Could you check a few things on this drawing? It's one solid part, dimensions in mm from its lowest x, y, z. A direction names the side the tool comes from. Give positions to 0.01 mm unless a question says otherwise; leave off trailing zeros.
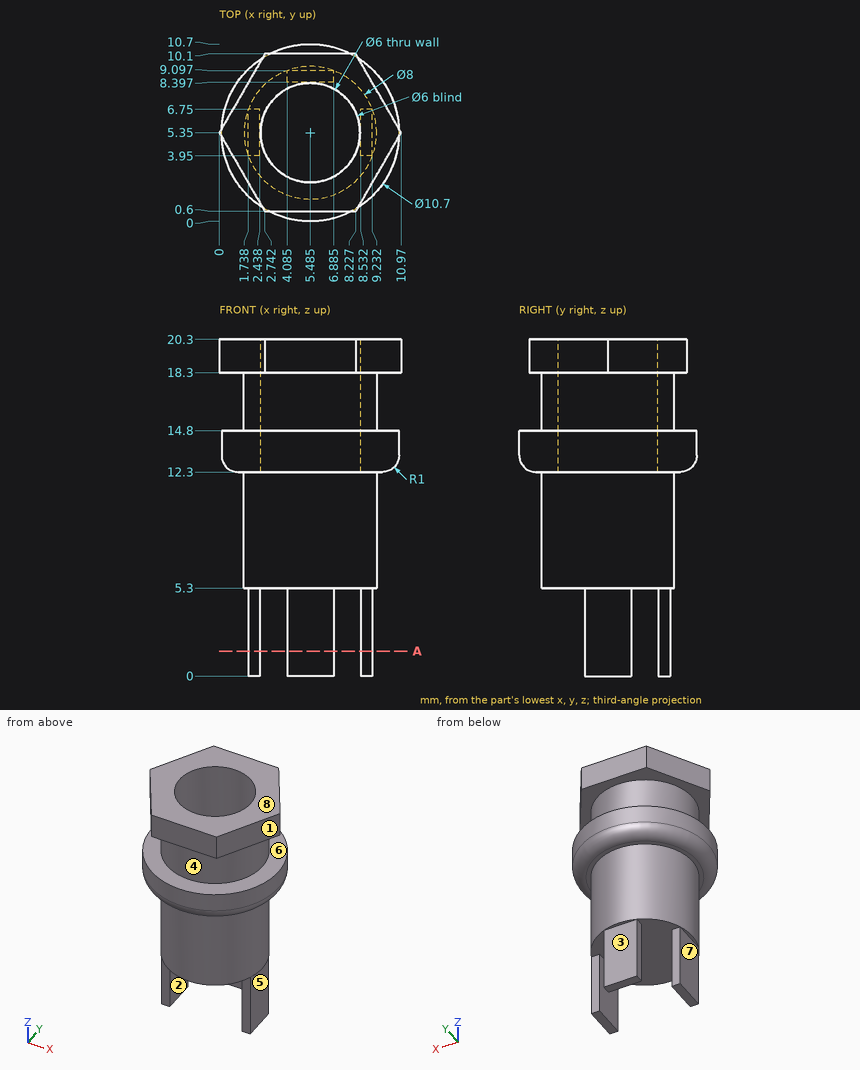
Item 1: For pin 1 (1.6 mm diameter, centred on x = 4.5, z = 19, fed in from +Y); pin 2 (0.6 mm diameter, centred on x = 2, z = 2, fed in from -Y); pin 3 (0.6 mm diameter, centred on x = 9, z = 3.5, fed in from +Y); pin 4 (5.5 mm diameter, centred on x = 5.5, y = 7, fed in from +Z), each with a flat end and sliding along its axis, tell me the tip position at first contact or that it passes through.
Findings:
pin 1: stops at y = 10.1
pin 2: stops at y = 3.95
pin 3: stops at y = 6.75
pin 4: stops at z = 20.3
Item 2: We'd pull the mould along Z, two halves only. Please class the marked faces 6, 7 and 8: +Z half, -Z half, draft (parallel to the pull), parting line (faces both ways), or undercut.
Findings:
face 6: undercut
face 7: draft
face 8: +Z half
Item 3: Imagine slicing it at A-A on z = 1.5. Give the number of separate pieces and of enclosed holes in the cut face.
Findings:
separate pieces: 3
enclosed holes: 0
Item 4: Please list where these lines run through material, in increasing order: line 1 along Z through (x, y) = (4.5, 1.25); line 2 along Z through (x, y) = (7.25, 4.5); line 3 along Y through (x, z) = (5.25, 4).
Findings:
line 1: z = 12.3 to 14.8, 18.3 to 20.3
line 2: z = 5.3 to 12.3
line 3: y = 8.4 to 9.1
Item 5: For the marked faces 1, 2, 3, 4 and 5, which set-ups out of +Z, -Z, +X, -X, +Y, -Y let a thin tool reach every point of the face, with its end or its side?
Findings:
face 1: +Z, +X, -Y
face 2: -Z, +Y, -Y
face 3: -Z, +X, -X, +Y
face 4: none
face 5: -Z, +X, +Y, -Y
